Check sheet for the drawn part. Datum: minimum x, y, z corner. Units: mm. Round coordinates to 2 decimals unless told otherwise and drop trailing zeros. Write each loop counter-clockwise with the first axis right and the second up, starting at its lowest first coordinate (ties: lowest second). Pieces come first, ordered by that corner, then holes. Notation, with made-up numbers: (-35.75, 16) -> (-10.75, 16) arc R5 cw to (-10.75, 20) -> close; hole circle Ø9 at (60.5, 16.25). An arc over 180 degrees is marked (long way). Use a Markdown table: item, result.
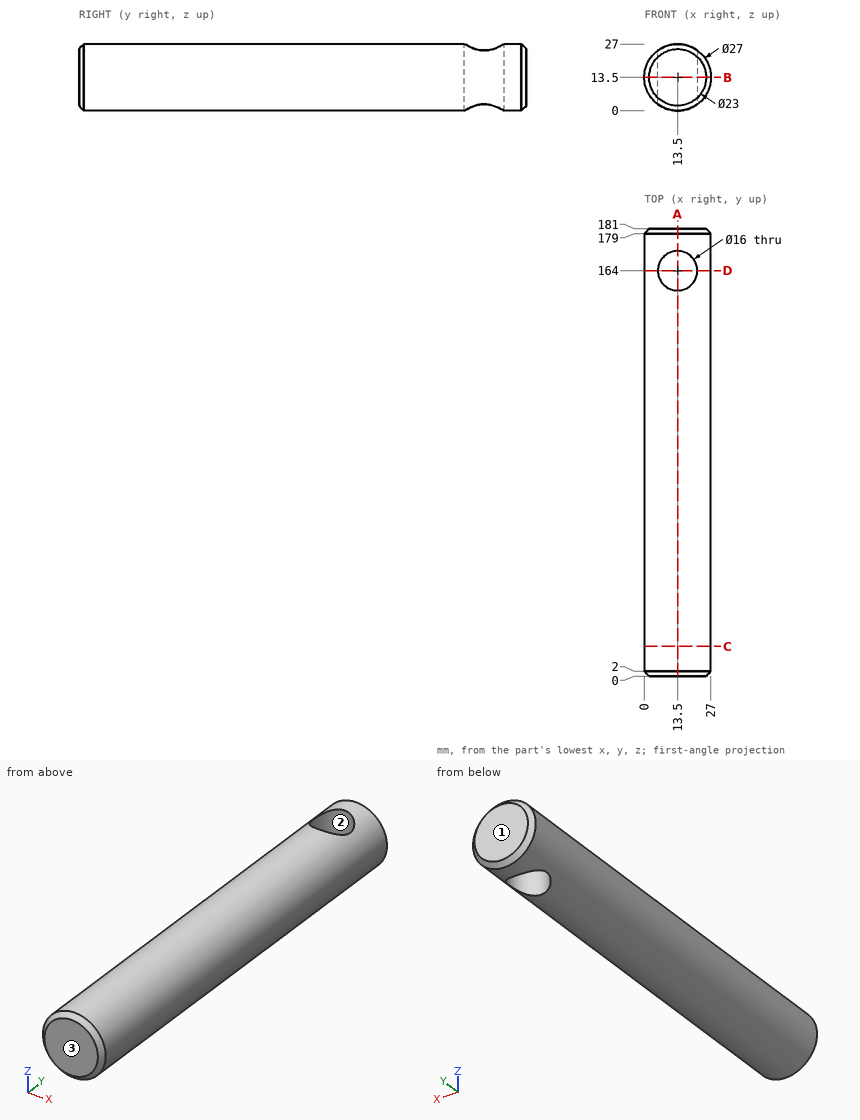
(1) Section check D-D on y = 164. Record the cut outline in (x, z).
A:
| item | result |
|---|---|
| outline | (5.5, 2.63) -> (5.5, 24.37) arc R13.5 ccw to start; (21.5, 2.63) arc R13.5 ccw to (21.5, 24.37) -> close |
(2) Section check B-B on z = 13.5. Record the cut outline in (x, y).
A:
| item | result |
|---|---|
| outline | (0, 2) -> (2, 0) -> (25, 0) -> (27, 2) -> (27, 179) -> (25, 181) -> (2, 181) -> (0, 179) -> close; hole circle Ø16 at (13.5, 164) |
(3) Gauge pin test, flat ends, axial feed: pin 1 Ø6 at (y, z) = (89, 7) entering from +X; pin 2 Ø1.5 at (x, y) = (21, 163) entering from -Z; pin 3 Ø14.5 at (x, y) = (13.5, 164) entering from -Z; pin 4 Ø10 at (x, y) = (5.5, 114.5) entering from +Z. Record the tip position at first contact, or that the pin passes through.
A:
| item | result |
|---|---|
| pin 1 | stops at x = 26.54 |
| pin 2 | stops at z = 2.5 |
| pin 3 | passes through |
| pin 4 | stops at z = 26.66 |
(4) Section check C-C on y = 12. Record the cut outline in (x, z).
A:
| item | result |
|---|---|
| outline | circle Ø27 at (13.5, 13.5) |
(5) Section check A-A on x = 13.5. Record the cut outline in (y, z), plus the area to 3 significant figures.
A:
| item | result |
|---|---|
| outline | (0, 2) -> (2, 0) -> (156, 0) -> (156, 27) -> (2, 27) -> (0, 25) -> close; (172, 0) -> (179, 0) -> (181, 2) -> (181, 25) -> (179, 27) -> (172, 27) -> close |
| area | 4,450 mm2 |
(6) Thickness scan on line 1 (Y direction, x = 13.5, z = 19); line 2 (Y direction, x = 20.25, z = 3.5); line 3 (X direction, y = 164, z = 8.25). Record the ranges inside material, lowest first.
A:
| item | result |
|---|---|
| line 1 | y = 0 to 156, 172 to 181 |
| line 2 | y = 0.56 to 159.71, 168.29 to 180.44 |
| line 3 | x = 1.06 to 5.5, 21.5 to 25.94 |
(7) Release check for a two-part mould opening along Y. For the marked faces 1, 2 and 3 record: +Y half, -Y half, draft (parallel to the pull), parting line (faces both ways), or undercut.
A:
| item | result |
|---|---|
| face 1 | +Y half |
| face 2 | undercut |
| face 3 | -Y half |
